Design review of the part shown in the three views and the two pictorial views. Dimensions are in mm from the part's minimum x, y and z. Round coordinates to 2 decimals unless told otherwise and drop trailing zeros. Order: outer loops, then holes, each group sorted by start corner. A loop starts at its lowest first (then second) coordinate and runs counter-clockwise, first axis right, second up. Notation, with made-up numbers: M -14,0 L 29,0 A14 ccw 29,6 Z; hole C -31,18.5 d10. An arc over 180 degrees is marked long. Use a Markdown table: item, result. Add a question column.
(1) Take a section at B-B (z = 8). Write out the cut boundary in (x, y).
(2) Take a section at A-A (x = 35). Write out the cut boundary in (y, z).
(3) Take a section at C-C (y = 3.05). Write out the cut boundary in (x, z).
(4) Take a section at D-D (x = 8.5). Write out the cut boundary in (y, z).
(5) To check wall thickness, follow probe 1 along X at (y, z) = (1.8, 8); probe 2 along Z at (x, y) = (7, 1.3); probe 3 along Z at (x, y) = (33, 2.1). State the ranges of each line that lie inside material, in increasing order. Write a range as from..to.
(6) The part is to be moulded in two halves that separate along Z. For the marked faces 1, 2 and 3, say which applies: released by +Z, released by -Z, zero draft, split by the parting line, or undercut.
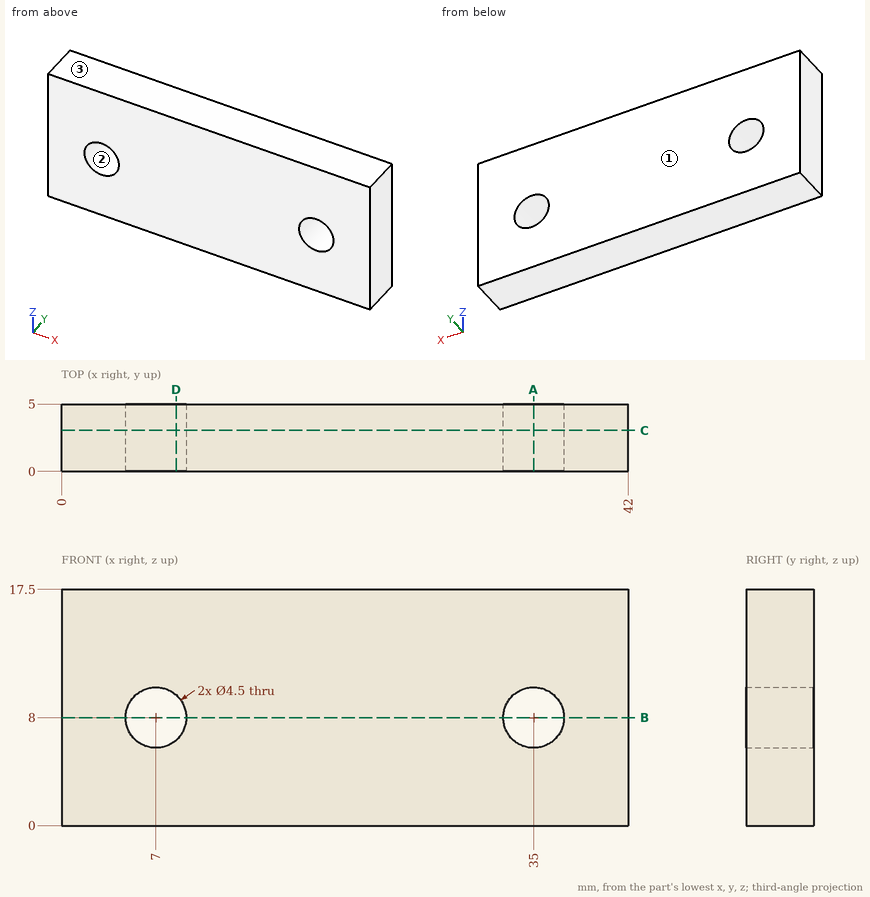
Verdict:
| question | item | result |
|---|---|---|
| 1 | outline | M 0,0 L 4.75,0 L 4.75,5 L 0,5 Z; M 9.25,0 L 32.75,0 L 32.75,5 L 9.25,5 Z; M 37.25,0 L 42,0 L 42,5 L 37.25,5 Z |
| 2 | outline | M 0,0 L 5,0 L 5,5.75 L 0,5.75 Z; M 0,10.25 L 5,10.25 L 5,17.5 L 0,17.5 Z |
| 3 | outline | M 0,0 L 42,0 L 42,17.5 L 0,17.5 Z; hole C 7,8 d4.5; hole C 35,8 d4.5 |
| 4 | outline | M 0,0 L 5,0 L 5,6.32 L 0,6.32 Z; M 0,9.68 L 5,9.68 L 5,17.5 L 0,17.5 Z |
| 5 | probe 1 | x = 0..4.75, 9.25..32.75, 37.25..42 |
| 5 | probe 2 | z = 0..5.75, 10.25..17.5 |
| 5 | probe 3 | z = 0..6.97, 9.03..17.5 |
| 6 | face 1 | zero draft |
| 6 | face 2 | undercut |
| 6 | face 3 | released by +Z |
